Build history of the part. All positions in model axes, mm. A direction names the side the tool comes from. Round coordinates to 2 decimals unless told otherwise and drop trailing zeros. Write each loop counter-clockwise with the first axis right and the second up, starting at its lowest first coordinate (ties: lowest second). Pieces come first, ordered by that corner, then holes. Notation, with made-up numbers: (-15, 26) -> (-1, 26) arc R7 ccw to (-1, 35) -> close; hole circle Ø4 at (9, 5.25). An arc over 180 degrees is marked (long way). One line per question, with ' | ' between items.
from build123d import *

# Parameters (mm, degrees)
SKETCH1_W                = 26
SKETCH1_H                = 53
SKETCH1_W_2              = 20
SKETCH1_H_2              = 10
BOSS_EXTRUDE1_DEPTH      = 5
SKETCH2_W                = 31
SKETCH2_H                = 59
SKETCH2_W_2              = 26
SKETCH2_H_2              = 53
BOSS_EXTRUDE2_DEPTH      = 10
SKETCH3_W                = 31
SKETCH3_H                = 59
BOSS_EXTRUDE3_DEPTH      = 3
CHAMFER1_SIZE            = 0.5
CHAMFER1_SIZE2           = 7.150333128
SKETCH10_W               = 7
SKETCH10_H               = 15
SKETCH10_R               = 2.25
BOSS_EXTRUDE7_DEPTH      = 10
BOSS_EXTRUDE9_DEPTH      = 3
BOSS_EXTRUDE9_DEPTH_BACK = 12
SKETCH12_R               = 1.75
CUT_EXTRUDE4_DEPTH       = 30.54863335
SKETCH13_W               = 7
SKETCH13_H               = 3.8
CUT_EXTRUDE5_DEPTH       = 10


with BuildPart() as part:
    # Sketch1 → Boss-Extrude1 (new body)
    with BuildSketch(Plane(origin=(0, 0, 0), x_dir=(1, 0, 0), z_dir=(0, 1, 0))):
        with Locations((-13, 26.5)):
            Rectangle(SKETCH1_W, SKETCH1_H)
        with Locations((-13, 27)):
            Rectangle(SKETCH1_W_2, SKETCH1_H_2, mode=Mode.SUBTRACT)
        with Locations((-13, 43)):
            Rectangle(SKETCH1_W_2, SKETCH1_H_2, mode=Mode.SUBTRACT)
        with Locations((-13, 11)):
            Rectangle(SKETCH1_W_2, SKETCH1_H_2, mode=Mode.SUBTRACT)
    extrude(amount=BOSS_EXTRUDE1_DEPTH)

    # Sketch2 → Boss-Extrude2 (add)
    with BuildSketch(Plane(origin=(0, 5, 0), x_dir=(1, 0, 0), z_dir=(0, 1, 0))):
        with Locations((-13, 26.5)):
            Rectangle(SKETCH2_W, SKETCH2_H)
        with Locations((-13, 26.5)):
            Rectangle(SKETCH2_W_2, SKETCH2_H_2, mode=Mode.SUBTRACT)
    extrude(amount=-BOSS_EXTRUDE2_DEPTH)

    # Sketch3 → Boss-Extrude3 (add)
    with BuildSketch(Plane(origin=(0, 5, 0), x_dir=(1, 0, 0), z_dir=(0, 1, 0))):
        with Locations((-13, 26.5)):
            Rectangle(SKETCH3_W, SKETCH3_H)
    extrude(amount=BOSS_EXTRUDE3_DEPTH)

    # Chamfer1
    chamfer1_edges = [part.edges().sort_by_distance(p)[0] for p in [
        (-28.5, -5, -26.5),
        (2.5, -5, -26.5),
    ]]
    chamfer1_side = [part.faces().sort_by_distance(p)[0] for p in [
        (-13, -5, -55.333516692),
    ]]
    chamfer(chamfer1_edges, length=CHAMFER1_SIZE, length2=CHAMFER1_SIZE2, reference=chamfer1_side[0])

    # Sketch10 → Boss-Extrude7 (add)
    with BuildSketch(Plane(origin=(0, 8, 0), x_dir=(1, 0, 0), z_dir=(0, 1, 0))):
        with Locations((6, 4.5)):
            Rectangle(SKETCH10_W, SKETCH10_H)
        with Locations((5, 5)):
            Circle(SKETCH10_R, mode=Mode.SUBTRACT)
        with Locations((-32, 4.5)):
            Rectangle(SKETCH10_W, SKETCH10_H)
        with Locations((-31, 5)):
            Circle(SKETCH10_R, mode=Mode.SUBTRACT)
    extrude(amount=-BOSS_EXTRUDE7_DEPTH)

    # Sketch11 → Boss-Extrude9 (add, two sides)
    with BuildSketch(Plane.XY) as boss_extrude9_sk:
        with BuildLine():
            Line((-13.74863335, 28.198986818), (-12.25136665, 28.198986818))
            Line((-12.25136665, 28.198986818), (-12.25136665, 33.909462138))
            ThreePointArc((-12.25136665, 33.909462138), (-8.80136665, 38), (-12.25136665, 42.090537862))
            Line((-12.25136665, 42.090537862), (-12.25136665, 50.4))
            Line((-12.25136665, 50.4), (-5.95136665, 50.4))
            Line((-5.95136665, 50.4), (-5.95136665, 18))
            Line((-5.95136665, 18), (1.04863335, 11))
            Line((1.04863335, 11), (1.04863335, 8))
            Line((1.04863335, 8), (-27.04863335, 8))
            Line((-27.04863335, 8), (-27.04863335, 11))
            Line((-27.04863335, 11), (-20.04863335, 18))
            Line((-20.04863335, 18), (-20.04863335, 50.4))
            Line((-20.04863335, 50.4), (-13.74863335, 50.4))
            Line((-13.74863335, 50.4), (-13.74863335, 42.090537862))
            ThreePointArc((-13.74863335, 42.090537862), (-17.19863335, 38), (-13.74863335, 33.909462138))
            Line((-13.74863335, 33.909462138), (-13.74863335, 28.198986818))
        make_face()
    extrude(amount=BOSS_EXTRUDE9_DEPTH)
    extrude(boss_extrude9_sk.sketch, amount=-BOSS_EXTRUDE9_DEPTH_BACK)

    # Sketch12 → Cut-Extrude4 (cut, through all)
    with BuildSketch(Plane(origin=(-5.95136665, 0, 0), x_dir=(0, 0, -1), z_dir=(1, 0, 0))):
        with Locations((4.5, 46.4)):
            Circle(SKETCH12_R)
    extrude(amount=-CUT_EXTRUDE4_DEPTH, mode=Mode.SUBTRACT)

    # Sketch13 → Cut-Extrude5 (cut)
    with BuildSketch(Plane(origin=(0, 8, 0), x_dir=(1, 0, 0), z_dir=(0, 1, 0))):
        with Locations((-32, 10.1)):
            Rectangle(SKETCH13_W, SKETCH13_H)
    extrude(amount=-CUT_EXTRUDE5_DEPTH, mode=Mode.SUBTRACT)


solid = part.part
(1) Slice it at B-B (y = 46.4). Write the cut outline in (x, z).
Calculated:
outline: (-20.05, -12) -> (-13.75, -12) -> (-13.75, -6.25) -> (-20.05, -6.25) -> close; (-20.05, -2.75) -> (-13.75, -2.75) -> (-13.75, 3) -> (-20.05, 3) -> close; (-12.25, -12) -> (-5.95, -12) -> (-5.95, -6.25) -> (-12.25, -6.25) -> close; (-12.25, -2.75) -> (-5.95, -2.75) -> (-5.95, 3) -> (-12.25, 3) -> close
(2) Wall check: line 1 (X direction, y = 5.25, z = -5); line 2 (Z direction, x = -31, y = 1); line 3 (Z direction, x = 5, y = 3.25). Give the ranges that are in metal, low to high. Write a range as from..to.
Calculated:
line 1: -35.5..-33.25, -28.75..2.75, 7.25..9.5 | line 2: -8.2..-7.25, -2.75..3 | line 3: -12..-7.25, -2.75..3
(3) Slice it at D-D (x = -31). Write the cut outline in (y, z), then the cut area to 3 significant figures.
Calculated:
outline: (-2, -8.2) -> (8, -8.2) -> (8, -7.25) -> (-2, -7.25) -> close; (-2, -2.75) -> (8, -2.75) -> (8, 3) -> (-2, 3) -> close | area: 67.0 mm2
(4) Mould opens along Y. For faces 1 (the flat face through (2.5, 5, -34)), 2 (the flat face through (-9, 50.4, -4)), 3 (the cylindrical face through (-8.802, 37.919, -4.395)) say: pulls with the +Y half, pulls with the -Y half, needs draft (parallel to the pull), parting line crosses it, or undercut.
Calculated:
face 1: needs draft | face 2: pulls with the +Y half | face 3: undercut
(5) Slice it at A-A (x = 5). Write the cut outline in (y, z).
Calculated:
outline: (-2, -12) -> (8, -12) -> (8, -7.25) -> (-2, -7.25) -> close; (-2, -2.75) -> (8, -2.75) -> (8, 3) -> (-2, 3) -> close
(6) Slice it at C-C (z = -40). Write the cut outline in (x, y), then the cut area to 3 significant figures.
Calculated:
outline: (-28.5, 2.15) -> (-28, -5) -> (-26, -5) -> (-26, 0) -> (-23, 0) -> (-23, 5) -> (-3, 5) -> (-3, 0) -> (0, 0) -> (0, -5) -> (2, -5) -> (2.5, 2.15) -> (2.5, 8) -> (-28.5, 8) -> close | area: 169 mm2
(7) 3-axis set-ups, long thin cutter, end or side, ignore diameter. For faces 4 (the flat face through (1.049, 10, -4)), 5 (the flat face through (-27.049, 9, -4)), 6 (the flat face through (-13.749, 31, -4)), 7 (the flat face through (-13, 2, -22)): which of +Z, -Z, +X, -X, +Y, -Y reach the whole face in a straight line?
Calculated:
face 4: +Z, -Z, +X, +Y | face 5: +Z, -Z, -X, +Y | face 6: +Z, -Z, +Y | face 7: -Y
(8) Drop flat-ended pins along their axis: pin 1 (5 mm diameter, centred on x = -15, z = -9.5, fed in from -Y); pin 2 (2.5 mm diameter, centred on y = -2.5, z = -36.5, fed in from +X); pin 3 (3 mm diameter, centred on x = 2.5, z = -49.5, fed in from +Y). Give the stop position or say it passes through.
Calculated:
pin 1: y = 5 | pin 2: x = 2.26 | pin 3: y = 8
